```python
from build123d import *

# Parameters (mm, degrees)
M8_TAPPED_HOLE1_D     = 6
M8_TAPPED_HOLE1_DEPTH = 9.75
FILLET1_R             = 5


with BuildPart() as part:
    # Sketch1 → Revolve1 (revolve)
    with BuildSketch(Plane(origin=(0, 0, 0), x_dir=(0, 0, -1), z_dir=(1, 0, 0))):
        Polygon((0, 0), (5, 0), (8.566874978, 9), (3.5, 14), (0, 14), align=None)
    revolve(axis=Axis((0, 0, 0), (0, 1, 0)))

    # M8 Tapped Hole1
    with Locations(Plane(origin=(0, 14, 0), x_dir=(1, 0, 0), z_dir=(0, 1, 0))):
        with Locations((0, 0)):
            Hole(M8_TAPPED_HOLE1_D / 2, depth=M8_TAPPED_HOLE1_DEPTH)

    # Fillet1
    fillet1_edges = [part.edges().sort_by_distance(p)[0] for p in [
        (0, 9, 8.566874978),
    ]]
    fillet(fillet1_edges, radius=FILLET1_R)


solid = part.part
```
Design review of the part built by this model. Coordinates are the model's own, in mm. A direction names the side the tool comes from. Round coordinates to 2 decimals unless told otherwise and drop trailing zeros. Put each result on its own line as item: value.
Q1. Draft analysis for pull direction X (two halves, no side actions). For faces 1 (the face through (3, 9, 0)), 2 (the face through (0, 0, 0)), 3 (the face through (-1.62, 1.03, -5.16)), state which applies: released by +X, released by -X, zero draft, split by the parting line, or undercut.
Reported:
face 1: undercut
face 2: zero draft
face 3: split by the parting line
Q2. To check wall thickness, follow line 1 (Y direction, x = 2.5, z = 1); line 2 (X direction, y = 5.25, z = 1.25); line 3 (Z direction, x = 0, y = 11.5). State the ranges of each line that lie inside material, in increasing order.
Reported:
line 1: 0 to 4.25
line 2: -6.97 to -2.73, 2.73 to 6.97
line 3: -6.03 to -3, 3 to 6.03
Q3. Machinability: for faces 4 (the face through (0, 4.25, 0)), 5 (the face through (-1, 14, -3)), which of the approach directions +Z, -Z, +X, -X, +Y, -Y give a long, thin tool a straight path to every point of the face, cutting with its end or side? Answer none if there is none.
Reported:
face 4: +Y
face 5: +Z, -Z, +X, -X, +Y
Q4. Insertion check: pin 1 Ø3 at (y, z) = (9, 4.5) entering from +X; pin 2 Ø1 at (x, y) = (3, 7) entering from -Z; pin 3 Ø1.5 at (x, y) = (1.5, 7) entering from +Z. Each pin has a flat end and moves straight along its axis. Give the tip position at first contact, or say it passes through.
Reported:
pin 1: x = 6.99
pin 2: z = -7.23
pin 3: z = 7.64
